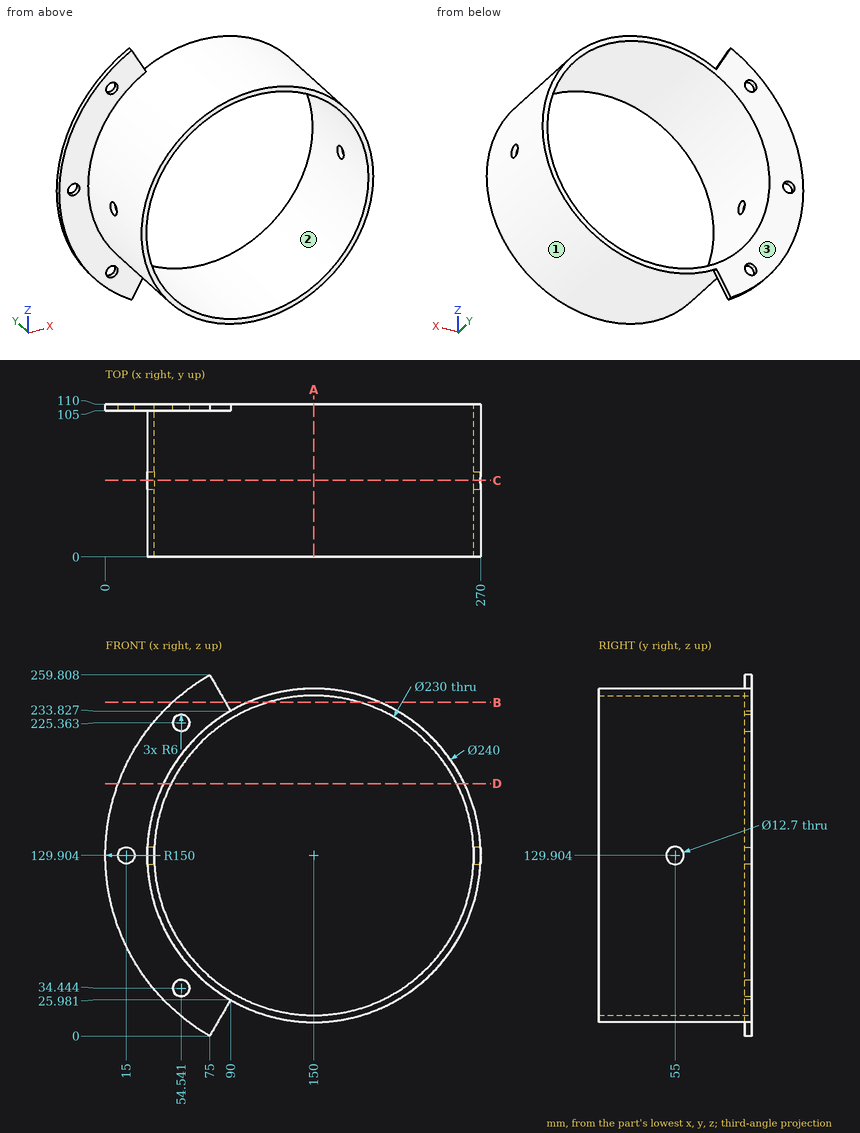
Here's the drawing with two shaded views (mm, measured from the low corner). I have some questions. Coordinates: 2 decimals unless noted, no trailing zeros. Loops run counter-clockwise (first coordinate to the right, second up) from the corner with the lowest first, then second, coordinate; pieces in that order, holes last. Notation, with made-up numbers: (77.25, 4.5) -> (130.25, 4.5) arc R20 cw to (130.25, 34.5) -> close; hole circle Ø7 at (74.5, 16.5). An arc over 180 degrees is marked (long way). Put each result on its own line as item: value. Start each with the question number.
Q1. I want a section at B-B (z = 240). Write out the boundary of the cut face in (x, y), plus the area to 3 significant figures.
Q2. I'm going to push flat-ended pins straight in: P1, Ø1, axis at y = 55, z = 110.5, coming from the +X side; P2, Ø4, axis at x = 174.5, y = 22.5, coming from the -Z side; P3, Ø5, axis at y = 92.5, z = 202, coming from the +X side. Where does each tip first touch, or does it pass through?
Q3. Thinking about a two-plate mould opening in Z: for the marked faces 1, 2 and 3, which applies, pulls with the +Z half, pulls with the -Z half, needs draft (parallel to the pull), parting line crosses it, or undercut?
Q4. I want a section at D-D (z = 181.5). Write out the boundary of the cut face in (x, y) (1 decimal).
Q5. I want a section at A-A (x = 150). Write out the boundary of the cut face in (y, z), plus the area to 3 significant figures.
Q6. I want a section at C-C (y = 55). Write out the boundary of the cut face in (x, z) (1 decimal).
Q7. If I drill on line 1 (X direction, y = 28.5, z = 84); line 2 (X direction, y = 19.5, z = 211.5) (1 decimal); line 3 (Z direction, x = 178.5, y = 47.5), over which ranges is the centre line in solid material (lowest first)? Write a range as [from, to].
Taken from the geometry:
1. outline: (48.12, 105) -> (86.44, 105) -> (86.44, 110) -> (48.12, 110) -> close; (102.26, 0) -> (116.78, 0) -> (116.78, 110) -> (102.26, 110) -> close; (183.22, 0) -> (197.74, 0) -> (197.74, 110) -> (183.22, 110) -> close
1. area: 3,380 mm2
2. P1: stops at x = 268.5
2. P2: stops at z = 12.03
2. P3: stops at x = 247.76
3. face 1: parting line crosses it
3. face 2: undercut
3. face 3: needs draft
4. outline: (9.2, 105) -> (41.7, 105) -> (41.7, 0) -> (47.2, 0) -> (47.2, 110) -> (9.2, 110) -> close; (252.8, 0) -> (258.3, 0) -> (258.3, 110) -> (252.8, 110) -> close
5. outline: (0, 9.9) -> (110, 9.9) -> (110, 14.9) -> (0, 14.9) -> close; (0, 244.9) -> (110, 244.9) -> (110, 249.9) -> (0, 249.9) -> close
5. area: 1,100 mm2
6. outline: (30.2, 123.6) arc R120 ccw to (269.8, 123.6) -> (264.8, 123.6) arc R115 cw to (35.2, 123.6) -> close; (30.2, 136.3) -> (35.2, 136.3) arc R115 cw to (264.8, 136.3) -> (269.8, 136.3) arc R120 ccw to start
7. line 1: x = [39.13, 44.56], [255.44, 260.87]
7. line 2: x = [62, 69], [231, 238]
7. line 3: z = [13.34, 18.49], [241.32, 246.47]
